The listing builds one solid part. Answer for the finished solid, in the listing's coordinates (mm). Round coordinates to 2 decimals unless told otherwise and drop trailing zeros. Loops run counter-clockwise (first coordinate to the right, second up) from the corner with the lowest first, then second, coordinate; pieces in that order, holes last. Notation, with made-up numbers: M 88.25,-16 L 125.25,-16 A17 cw 125.25,11 Z; hole C -19.75,1 d9. An arc over 180 degrees is marked long. Answer as a JSON object with one key per item and string values.
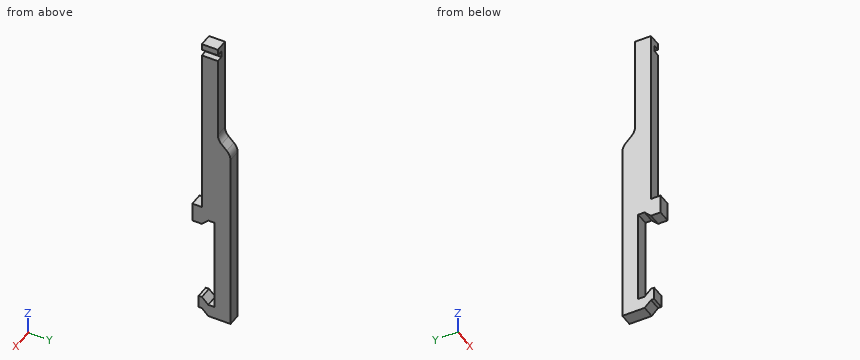
```python
from build123d import *

# Parameters (mm, degrees)
SKETCH_1_W          = 16
SKETCH_1_H          = 2.5
EXTRUDE_1_DEPTH     = 2
FILLET_1_R          = 2
SKETCH_2_W          = 1
SKETCH_2_H          = 1
CUT_EXTRUDE_1_DEPTH = 49.207883173


with BuildPart() as part:
    # Эскиз1 → Бобышка-Вытянуть1 (new body)
    with BuildSketch(Plane(origin=(0, 0, 0), x_dir=(0, 0, -1), z_dir=(1, 0, 0))):
        Polygon((48, 1), (48, 4.5), (29, 4.5), (18, 4.5), (16, 2.5), (16, 0), (29, 0), (29, -1.5), (32, -1.5), (32, 0), (31, 1), (31, 2), (46, 2), (46, 1), (45, 0), (45, -0.5), (47, -0.5), (47, 0), align=None)
        with Locations((8, 1.25)):
            Rectangle(SKETCH_1_W, SKETCH_1_H)
    extrude(amount=EXTRUDE_1_DEPTH)

    # Скругление1
    fillet_1_edges = [part.edges().sort_by_distance(p)[0] for p in [
        (1, 2.5, -16),
        (1, 4.5, -18),
    ]]
    fillet(fillet_1_edges, radius=FILLET_1_R)

    # Эскиз2 → Вырез-Вытянуть1 (cut, through all)
    with BuildSketch(Plane(origin=(0, 2.5, 0), x_dir=(1, 0, 0), z_dir=(0, 1, 0))):
        with Locations((1.5, 1.5)):
            Rectangle(SKETCH_2_W, SKETCH_2_H)
    extrude(amount=-CUT_EXTRUDE_1_DEPTH, mode=Mode.SUBTRACT)


solid = part.part
```
Item 1: Straight lines are drawn through the part: line 1 (Z direction, x = 1.8, y = 1.1); line 2 (Z direction, x = 0.75, y = 1.4); line 3 (Z direction, x = 1.55, y = 0.5). For each, find the intervals that lie inside material, in ascending order.
Values follow:
{"line 1": "-48 to -46, -31 to -2, -1 to 0", "line 2": "-48 to -46, -31 to 0", "line 3": "-47.5 to -45.5, -31.5 to -2, -1 to 0"}
Item 2: The part is cut by section C-C (z = -24.5). Give the vertices of the cut face in (x, y).
Values follow:
{"outline": "M 0,0 L 2,0 L 2,4.5 L 0,4.5 Z"}
Item 3: The part is cut by section B-B (z = -31.5). Give the vertices of the cut face in (x, y), then the cut area to 3 significant figures.
Values follow:
{"outline": "M 0,-1.5 L 2,-1.5 L 2,0.5 L 0,0.5 Z; M 0,2 L 2,2 L 2,4.5 L 0,4.5 Z", "area": "9.00 mm^2"}
Item 4: The part is cut by section A-A (y = 1.4). Give the vertices of the cut face in (x, z).
Values follow:
{"outline": "M 0,-48 L 2,-48 L 2,-46 L 0,-46 Z; M 0,-31 L 2,-31 L 2,-2 L 1,-2 L 1,-1 L 2,-1 L 2,0 L 0,0 Z"}
Item 5: Flat-ended cylindrical pins translate along their axes: P1, Ø0.8, axis at y = 1, z = -1.5, coming from the +X side; P2, Ø1, axis at x = 1.5, z = -10, coming from the -Y side; P3, Ø0.6, axis at x = 1, z = -35, coming from the -Y side; P4, Ø0.8, axis at x = 1.5, y = 1, coming from the +Z side. Find the tip coordinate at first contact, or state that the pin passes through.
Values follow:
{"P1": "x = 1", "P2": "y = 0", "P3": "y = 2", "P4": "z = 0"}
